from build123d import *

# Parameters (mm, degrees)
EXTRUDE_1_DEPTH     = 6.5
SKETCH_2_R          = 0.4
EXTRUDE_2_DEPTH     = 0.2
SKETCH_3_R          = 3.5
EXTRUDE_3_DEPTH     = 5
SKETCH_4_R          = 3
EXTRUDE_5_DEPTH     = 10
SKETCH_5_W          = 6.52724622
SKETCH_5_H          = 2.89226862
CUT_EXTRUDE_1_DEPTH = 7
CHAMFER_1_SIZE      = 0.5
SKETCH_6_R          = 3.145240335
SKETCH_6_R_2        = 2.148425486
CUT_EXTRUDE_2_DEPTH = 0.5
SWEEP_START         = -1.25
SWEEP_12_DEPTH      = 2.5
SWEEP_START_2       = -1.200661392
SWEEP_13_DEPTH      = 2.5
SKETCH_13_W         = 0.8
SKETCH_13_H         = 0.1
SKETCH_14_W         = 0.8
SKETCH_14_H         = 0.1
FILLET_1_R          = 0.4
FILLET_2_R          = 1


# Read off the part's stored shape, not the designer's step: По траектории12, По траектории13
# Some blends are built 0.0001 mm under size
with BuildPart() as part:
    # Эскиз1 → Бобышка-Вытянуть1 (new body)
    with BuildSketch(Plane.XY):
        with BuildLine():
            Line((-5.75, 6.7), (5.75, 6.7))
            ThreePointArc((5.75, 6.7), (6.103553391, 6.553553391), (6.25, 6.2))
            Line((6.25, 6.2), (6.25, -6.2))
            ThreePointArc((6.25, -6.2), (6.103553391, -6.553553391), (5.75, -6.7))
            Line((5.75, -6.7), (-5.75, -6.7))
            ThreePointArc((-5.75, -6.7), (-6.103553391, -6.553553391), (-6.25, -6.2))
            Line((-6.25, -6.2), (-6.25, 6.2))
            ThreePointArc((-6.25, 6.2), (-6.103553391, 6.553553391), (-5.75, 6.7))
        make_face()
    extrude(amount=EXTRUDE_1_DEPTH)

    # Эскиз2 → Бобышка-Вытянуть2 (add)
    with BuildSketch(Plane.XY.offset(6.5)):
        with Locations((-4.6, 4.6)):
            Circle(SKETCH_2_R)
        with Locations((4.6, 4.6)):
            Circle(SKETCH_2_R)
        with Locations((4.6, -4.6)):
            Circle(SKETCH_2_R)
        with Locations((-4.6, -4.6)):
            Circle(SKETCH_2_R)
    extrude(amount=EXTRUDE_2_DEPTH)

    # Эскиз3 → Бобышка-Вытянуть3 (add)
    with BuildSketch(Plane.XY.offset(6.5)):
        Circle(SKETCH_3_R)
    extrude(amount=EXTRUDE_3_DEPTH)

    # Эскиз4 → Бобышка-Вытянуть5 (add)
    with BuildSketch(Plane.XY.offset(11.5)):
        Circle(SKETCH_4_R)
    extrude(amount=EXTRUDE_5_DEPTH)

    # Эскиз5 → Вырез-Вытянуть1 (cut)
    with BuildSketch(Plane.XY.offset(21.5)):
        with Locations((0, -2.94613431)):
            Rectangle(SKETCH_5_W, SKETCH_5_H)
    extrude(amount=-CUT_EXTRUDE_1_DEPTH, mode=Mode.SUBTRACT)

    # Фаска1
    chamfer_1_edges = [part.edges().sort_by_distance(p)[0] for p in [
        (-0.776457135, 2.897777479, 21.5),
    ]]
    chamfer(chamfer_1_edges, length=CHAMFER_1_SIZE)

    # Эскиз6 → Вырез-Вытянуть2 (cut)
    with BuildSketch(Plane.XY.offset(11.5)):
        Circle(SKETCH_6_R)
        Circle(SKETCH_6_R_2, mode=Mode.SUBTRACT)
    extrude(amount=CUT_EXTRUDE_2_DEPTH, mode=Mode.SUBTRACT)

    # По траектории12 outline → По траектории12 (add)
    with BuildSketch(Plane(origin=(0, 0, 0), x_dir=(1, 0, 0), z_dir=(0, 1, 0)).offset(SWEEP_START)):
        with BuildLine():
            Line((-5.85, 0), (-6.557222106, 1.597963985))
            add(Edge.make_bspline(
                [(-6.557222106, 1.597963985), (-6.632428218, 1.767891731), (-6.602440024, 1.979444008), (-6.482970147, 2.121775827)],
                knots=[0.400295136, 0.400295136, 0.400295136, 0.400295136, 0.527997483, 0.527997483, 0.527997483, 0.527997483], degree=3))
            Line((-6.482970147, 2.121775827), (-5.158247051, 3.7))
            Line((-5.158247051, 3.7), (-5.558247051, 3.7))
            Line((-5.558247051, 3.7), (-6.882970147, 2.121775827))
            add(Edge.make_bspline(
                [(-6.957222106, 1.597963985), (-7.032428218, 1.767891731), (-7.002440024, 1.979444008), (-6.882970147, 2.121775827)],
                knots=[0.400295136, 0.400295136, 0.400295136, 0.400295136, 0.527997483, 0.527997483, 0.527997483, 0.527997483], degree=3))
            Line((-6.957222106, 1.597963985), (-6.25, 0))
            Line((-6.25, 0), (-5.85, 0))
        make_face()
    extrude(amount=SWEEP_12_DEPTH)

    # По траектории13 outline → По траектории13 (add)
    with BuildSketch(Plane(origin=(0, 0, 0), x_dir=(1, 0, 0), z_dir=(0, 1, 0)).offset(SWEEP_START_2)):
        with BuildLine():
            Line((6.25, 0), (6.957222106, 1.597963985))
            add(Edge.make_bspline(
                [(6.957222106, 1.597963985), (7.032428218, 1.767891731), (7.002440024, 1.979444008), (6.882970147, 2.121775827)],
                knots=[0.400295136, 0.400295136, 0.400295136, 0.400295136, 0.527997483, 0.527997483, 0.527997483, 0.527997483], degree=3))
            Line((6.882970147, 2.121775827), (5.558247051, 3.7))
            Line((5.558247051, 3.7), (5.158247051, 3.7))
            Line((5.158247051, 3.7), (6.482970147, 2.121775827))
            add(Edge.make_bspline(
                [(6.557222106, 1.597963985), (6.632428218, 1.767891731), (6.602440024, 1.979444008), (6.482970147, 2.121775827)],
                knots=[0.400295136, 0.400295136, 0.400295136, 0.400295136, 0.527997483, 0.527997483, 0.527997483, 0.527997483], degree=3))
            Line((6.557222106, 1.597963985), (5.85, 0))
            Line((5.85, 0), (6.25, 0))
        make_face()
    extrude(amount=SWEEP_13_DEPTH)

    # По траектории14: sweep along a path in Эскиз15
    with BuildLine(Plane(origin=(0, 0, 0), x_dir=(0, 0, -1), z_dir=(1, 0, 0))) as sweep_14_path:
        Line((3.7, -7), (0, -7))
        ThreePointArc((0, -7), (-0.212132034, -6.912132034), (-0.3, -6.7))
    # Эскиз13 → По траектории14 (sweep)
    with BuildSketch(Plane(origin=(0, 0, 0), x_dir=(-1, 0, 0), z_dir=(0, 0, -1))):
        with Locations((2.5, -6.95)):
            Rectangle(SKETCH_13_W, SKETCH_13_H)
        with Locations((-2.5, -6.95)):
            Rectangle(SKETCH_13_W, SKETCH_13_H)
    sweep(path=sweep_14_path.line)

    # По траектории15: sweep along a path in Эскиз16
    with BuildLine(Plane(origin=(0, 0, 0), x_dir=(0, 0, -1), z_dir=(1, 0, 0))) as sweep_15_path:
        Line((3.344273236, 7.5), (0, 7.5))
        Line((0, 7.5), (-3, 7.5))
        ThreePointArc((-3, 7.5), (-3.176776695, 7.426776695), (-3.25, 7.25))
        Line((-3.25, 7.25), (-3.25, 6.7))
    # Эскиз14 → По траектории15 (sweep)
    with BuildSketch(Plane(origin=(0, 0, 0), x_dir=(-1, 0, 0), z_dir=(0, 0, -1))):
        with Locations((2.5, 7.45)):
            Rectangle(SKETCH_14_W, SKETCH_14_H)
        with Locations((0, 7.45)):
            Rectangle(SKETCH_14_W, SKETCH_14_H)
        with Locations((-2.5, 7.45)):
            Rectangle(SKETCH_14_W, SKETCH_14_H)
    sweep(path=sweep_15_path.line)

    # Скругление1
    fillet_1_edges = [part.edges().sort_by_distance(p)[0] for p in [
        (-2.9, -6.95, -3.7),
        (-2.1, -6.95, -3.7),
        (2.1, -6.95, -3.7),
        (2.9, -6.95, -3.7),
        (-2.9, 7.45, -3.344273236),
        (-2.1, 7.45, -3.344273236),
        (0.4, 7.45, -3.344273236),
        (-0.4, 7.45, -3.344273236),
        (2.1, 7.45, -3.344273236),
        (2.9, 7.45, -3.344273236),
    ]]
    fillet(fillet_1_edges, radius=FILLET_1_R - 0.0001)  # a hair under: the kernel refuses the full size

    # Скругление2
    # the kernel refuses this fillet: 1 mm, written as the material it takes off along each edge
    with BuildSketch(Plane(origin=(8.058247051, -1.200661392, -3.7), x_dir=(0, 0, 1), z_dir=(-1, 0, 0)), Plane(origin=(-2.658247051, -1.25, -3.7), x_dir=(0, 0, 1), z_dir=(-1, 0, 0))) as fillet_2_piece_1:
        with BuildLine():
            CenterArc((FILLET_2_R, FILLET_2_R), FILLET_2_R, 180, 90)
            Line((0, FILLET_2_R), (0, 0))
            Line((0, 0), (FILLET_2_R, 0))
        make_face()
    extrude(amount=5.4, mode=Mode.SUBTRACT)
    with BuildSketch(Plane(origin=(8.058247051, 1.299338608, -3.7), x_dir=(0, 0, 1), z_dir=(-1, 0, 0)), Plane(origin=(-2.658247051, 1.25, -3.7), x_dir=(0, 0, 1), z_dir=(-1, 0, 0))) as fillet_2_piece_2:
        with BuildLine():
            CenterArc((FILLET_2_R, -FILLET_2_R), FILLET_2_R, 90, 90)
            Line((0, -FILLET_2_R), (0, 0))
            Line((0, 0), (FILLET_2_R, 0))
        make_face()
    extrude(amount=5.4, mode=Mode.SUBTRACT)


solid = part.part
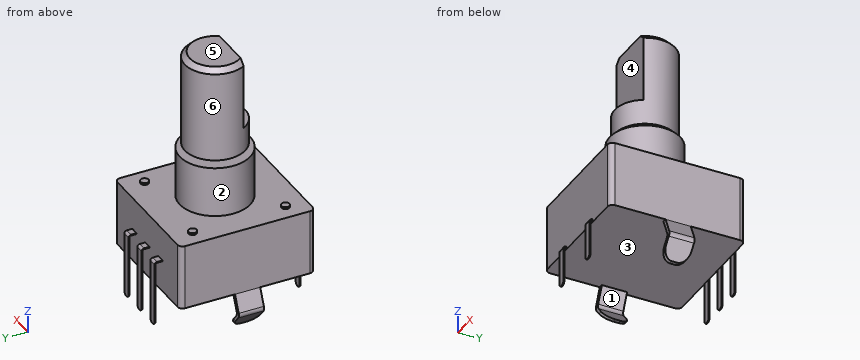
Could you check a few things on this model? Use its own coordinates, in mm. Face numbers are marked on the shaded views. A direction names the side the tool comes from. Coordinates: 2 decimals unless noted, no trailing zeros. Loops run counter-clockwise (first coordinate to the right, second up) from the corner with the lowest first, then second, coordinate; pieces in that order, holes last.
1. Imagine slicing it at B-B (x = -4.6). Please give me the cut outline in (y, z), and give its area (3 significant figures).
2. We'd pull the mould along Y, two halves only. Please class the marked faces 1, 2 and 3: released by +Y, released by -Y, zero draft, split by the parting line, or undercut.
3. Imagine slicing it at D-D (y = 5.75). Please give me the cut outline in (x, z), and give its area (4 significant figures).
4. Imagine slicing it at C-C (z = 14). Please give me the cut outline in (x, y).
5. For P1, Ø6, axis at y = -2.5, z = 4.5, coming from the +X side; P2, Ø4, axis at x = -0.5, z = 17, coming from the -Y side; P3, Ø5, axis at y = -3, z = 4, coming from the -X side; P4, Ø2, axis at x = 5, z = 12.5, coming from the +Y side, each with a flat end and sliding along its axis, tell me the tip position at first contact or that it passes through.
6. For the marked faces 4, 5 and 6, which set-ups out of +Z, -Z, +X, -X, +Y, -Y let a thin tool reach every point of the face, with its end or its side?
7. Imagine slicing it at A-A (y = -4.6). Please give me the cut outline in (x, z), and give its area (3 significant figures).
8. I need wall thicknesses on L1, parallel to Z at x = 5.75, y = -2.5; L2, parallel to Y at x = 5, z = 1.5; L3, parallel to X at y = 4.5, z = 2.5. Which ranges of each line are inside material? Lowest first, please.
Computed values:
1. outline: (-6.7, 0) - (6.7, 0) - (6.7, 6.5) - (5, 6.5) - (5, 6.7) - (4.2, 6.7) - (4.2, 6.5) - (-4.2, 6.5) - (-4.2, 6.7) - (-5, 6.7) - (-5, 6.5) - (-6.7, 6.5) - close
1. area: 87.4 mm2
2. face 1: zero draft
2. face 2: split by the parting line
2. face 3: undercut
3. outline: (-6.25, 0) - (6.25, 0) - (6.25, 6.5) - (-6.25, 6.5) - close
3. area: 81.25 mm2
4. outline: circle Ø6 at (0, 0)
5. P1: stops at x = 6.25
5. P2: stops at y = -1.5
5. P3: stops at x = -6.25
5. P4: passes through
6. face 4: +Z, +X, -X, -Y
6. face 5: +Z, +X, -X, +Y, -Y
6. face 6: +Z
7. outline: (-6.25, 0) - (6.25, 0) - (6.25, 6.5) - (5, 6.5) - (5, 6.7) - (4.2, 6.7) - (4.2, 6.5) - (-4.2, 6.5) - (-4.2, 6.7) - (-5, 6.7) - (-5, 6.5) - (-6.25, 6.5) - close
7. area: 81.6 mm2
8. L1: z = 0 to 6.5
8. L2: y = -6.7 to 6.7
8. L3: x = -6.25 to 6.25
